Geometry check sheet. Reference: the model listing, model coordinates, mm. Coordinates: 2 decimals unless noted, no trailing zeros. Loops run counter-clockwise (first coordinate to the right, second up) from the corner with the lowest first, then second, coordinate; pieces in that order, holes last. Notation, with made-up numbers: M -36,-2.5 L -12,-2.5 A23 cw -12,28.5 Z; hole C 73.25,-37 d11. An arc over 180 degrees is marked long. Use CSV: the item, a comma, the result in double quotes.
```python
from build123d import *

# Parameters (mm, degrees)
SKETCH1_R                = 1.5
BOSS_EXTRUDE1_DEPTH      = 2
CUT_EXTRUDE1_DEPTH       = 2
M3_CLEARANCE_HOLE1_D     = 3.4
M3_CLEARANCE_HOLE1_DEPTH = 10
M3_CLEARANCE_HOLE1_TIP   = 1.021463052
CUT_EXTRUDE4_DEPTH       = 10


with BuildPart() as part:
    # Sketch1 → Boss-Extrude1 (new body)
    with BuildSketch(Plane(origin=(0, 0, 0), x_dir=(1, 0, 0), z_dir=(0, 1, 0))):
        with BuildLine():
            Line((-31.856435644, 6.435643564), (-25, 75))
            Line((-25, 75), (25, 75))
            Line((25, 75), (31.856435644, 6.435643564))
            ThreePointArc((31.856435644, 6.435643564), (32.5, 0), (31.856435644, -6.435643564))
            Line((31.856435644, -6.435643564), (25, -75))
            Line((25, -75), (-25, -75))
            Line((-25, -75), (-31.856435644, -6.435643564))
            ThreePointArc((-31.856435644, -6.435643564), (-32.5, 0), (-31.856435644, 6.435643564))
        make_face()
        with Locations(Location((-20, 34.641016151, 0), (0, 0, 270))):
            Circle(SKETCH1_R, mode=Mode.SUBTRACT)
        with Locations(Location((20, 34.641016151, 0), (0, 0, 90))):
            Circle(SKETCH1_R, mode=Mode.SUBTRACT)
        with Locations(Location((20, -34.641016151, 0), (0, 0, 270))):
            Circle(SKETCH1_R, mode=Mode.SUBTRACT)
        with Locations(Location((-20, -34.641016151, 0), (0, 0, 90))):
            Circle(SKETCH1_R, mode=Mode.SUBTRACT)
    extrude(amount=BOSS_EXTRUDE1_DEPTH)

    # Sketch2 → Cut-Extrude1 (cut)
    with BuildSketch(Plane(origin=(0, 2, 0), x_dir=(1, 0, 0), z_dir=(0, 1, 0))):
        with BuildLine():
            Line((-15, 70), (15, 70))
            ThreePointArc((15, 70), (16.5, 68.5), (15, 67))
            Line((15, 67), (-15, 67))
            ThreePointArc((-15, 67), (-16.5, 68.5), (-15, 70))
        make_face()
        with BuildLine():
            Line((-15, -70), (15, -70))
            ThreePointArc((15, -70), (16.5, -68.5), (15, -67))
            Line((15, -67), (-15, -67))
            ThreePointArc((-15, -67), (-16.5, -68.5), (-15, -70))
        make_face()
        with BuildLine():
            Line((-15, 37), (15, 37))
            ThreePointArc((15, 37), (16.5, 38.5), (15, 40))
            Line((15, 40), (-15, 40))
            ThreePointArc((-15, 40), (-16.5, 38.5), (-15, 37))
        make_face()
        with BuildLine():
            Line((-15, -37), (15, -37))
            ThreePointArc((15, -37), (16.5, -38.5), (15, -40))
            Line((15, -40), (-15, -40))
            ThreePointArc((-15, -40), (-16.5, -38.5), (-15, -37))
        make_face()
        with BuildLine():
            Line((1.5, 25), (1.5, -25))
            ThreePointArc((1.5, -25), (0, -26.5), (-1.5, -25))
            Line((-1.5, -25), (-1.5, 25))
            ThreePointArc((-1.5, 25), (0, 26.5), (1.5, 25))
        make_face()
    extrude(amount=-CUT_EXTRUDE1_DEPTH, mode=Mode.SUBTRACT)

    # M3 Clearance Hole1
    with Locations(Plane(origin=(-22.5, 2, -22.5), x_dir=(0, 0, 1), z_dir=(0, 1, 0))):
        with Locations((0, 0), (0, 45), (45, 45), (45, 0)):
            Hole(M3_CLEARANCE_HOLE1_D / 2, depth=M3_CLEARANCE_HOLE1_DEPTH)
            with Locations((0, 0, -(M3_CLEARANCE_HOLE1_DEPTH + M3_CLEARANCE_HOLE1_TIP / 2))):  # 118° drill point
                Cone(0, M3_CLEARANCE_HOLE1_D / 2, M3_CLEARANCE_HOLE1_TIP, mode=Mode.SUBTRACT)

    # Sketch11 → Cut-Extrude4 (cut)
    with BuildSketch(Plane(origin=(0, 2, 0), x_dir=(1, 0, 0), z_dir=(0, 1, 0))):
        with BuildLine():
            Line((16.5, -46), (16.5, -61))
            ThreePointArc((16.5, -61), (15, -62.5), (13.5, -61))
            Line((13.5, -61), (13.5, -46))
            ThreePointArc((13.5, -46), (15, -44.5), (16.5, -46))
        make_face()
        with BuildLine():
            Line((-16.5, -46), (-16.5, -61))
            ThreePointArc((-16.5, -61), (-15, -62.5), (-13.5, -61))
            Line((-13.5, -61), (-13.5, -46))
            ThreePointArc((-13.5, -46), (-15, -44.5), (-16.5, -46))
        make_face()
        with BuildLine():
            Line((-16.5, 46), (-16.5, 61))
            ThreePointArc((-16.5, 61), (-15, 62.5), (-13.5, 61))
            Line((-13.5, 61), (-13.5, 46))
            ThreePointArc((-13.5, 46), (-15, 44.5), (-16.5, 46))
        make_face()
        with BuildLine():
            Line((16.5, 46), (16.5, 61))
            ThreePointArc((16.5, 61), (15, 62.5), (13.5, 61))
            Line((13.5, 61), (13.5, 46))
            ThreePointArc((13.5, 46), (15, 44.5), (16.5, 46))
        make_face()
    extrude(amount=-CUT_EXTRUDE4_DEPTH, mode=Mode.SUBTRACT)


solid = part.part
```
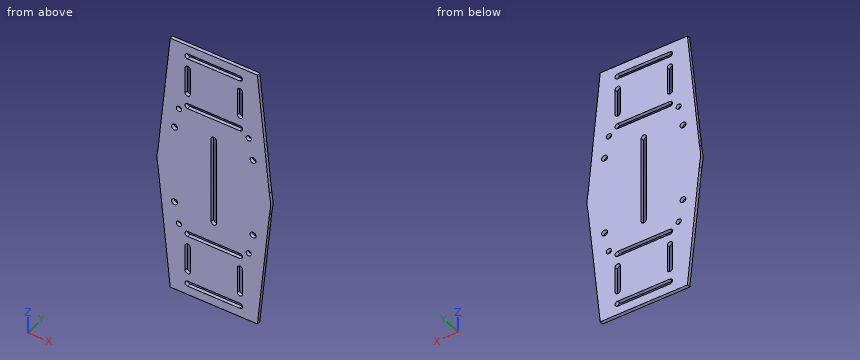
1. Gauge pin test, flat ends, axial feed: P1, Ø4, axis at x = -20, z = -34.64, coming from the -Y side; P2, Ø0.6, axis at y = 1.5, z = 51.5, coming from the +X side; P3, Ø0.6, axis at y = 1, z = 55.5, coming from the +X side; P4, Ø1, axis at y = 0.5, z = -57, coming from the -X side. Record the tip position at first contact, or that the pin passes through.
The answers:
P1,"y = 0"
P2,"x = 27.38"
P3,"x = 26.98"
P4,"x = -26.85"
2. Section check C-C, the plane z = 12.5. Record the cut outline in (x, y).
The answers:
outline,"M -31.25,0 L -1.5,0 L -1.5,2 L -31.25,2 Z; M 1.5,0 L 31.25,0 L 31.25,2 L 1.5,2 Z"
3. Section check A-A, the plane z = -10. Record the cut outline in (x, y), plus the area to 3 significant figures.
The answers:
outline,"M -31.5,0 L -1.5,0 L -1.5,2 L -31.5,2 Z; M 1.5,0 L 31.5,0 L 31.5,2 L 1.5,2 Z"
area,"120 mm^2"
4. Thickness scan on line 1 (Z direction, x = -11, y = 0.6); line 2 (X direction, y = 1.1, z = -60); line 3 (X direction, y = 0.2, z = -34). Record the ranges inside material, lowest first. Write a range as [from, to].
The answers:
line 1,"[-75, -70], [-67, -40], [-37, 37], [40, 67], [70, 75]"
line 2,"[-26.5, -16.5], [-13.5, 13.5], [16.5, 26.5]"
line 3,"[-29.1, -21.36], [-18.64, 18.64], [21.36, 29.1]"
5. Section check B-B, the plane x = -9.5. Record the cut outline in (y, z), plus the area to 3 significant figures.
The answers:
outline,"M 0,-75 L 2,-75 L 2,-70 L 0,-70 Z; M 0,-67 L 2,-67 L 2,-40 L 0,-40 Z; M 0,-37 L 2,-37 L 2,37 L 0,37 Z; M 0,40 L 2,40 L 2,67 L 0,67 Z; M 0,70 L 2,70 L 2,75 L 0,75 Z"
area,"276 mm^2"
